Autodesk Inventor part; units mm, degrees
ref_plane "作業平面1" through (14.45, -5.25, 10.5) normal (0, 0, 1) x (0, 1, 0)
ref_plane "YZ Plane" through (0, 0, 0) normal (1, 0, 0) x (0, 1, 0)
ref_plane "XZ Plane" through (0, 0, 0) normal (0, 1, 0) x (-1, 0, 0)
ref_plane "作業平面1" through (14.45, -5.25, 10.5) normal (0, 0, 1) x (0, 1, 0)
sketch "スケッチ1" plane through (14.45, -5.25, 10.5) normal (0, 0, 1) x (0, 1, 0)
  circle A0 centre (4.8, 4.5) radius 1.25
  circle A1 centre (4.8, 14.5) radius 1.25
  circle A2 centre (4.5, 225.5) radius 1.5
  circle A3 centre (4.5, 201.5) radius 1.5
  line L0 (9, 0) -> (0, 0)
  line L1 (9, 0) -> (9, 230)
  line L2 (0, 230) -> (9, 230)
  line L3 (0, 0) -> (0, 230)
  circle A4 centre (-11.4155, 9.5) radius 1.25
  circle A5 centre (4.8, 14.5) radius 4.6
  circle A6 centre (4.8, 4.5) radius 4.6
  circle A7 centre (-11.4155, 9.5) radius 4.25
  line L4 (9.4, 19.1) -> (-15.6655, 19.1)
  line L5 (-15.6655, 19.1) -> (-15.6655, -0.1)
  line L6 (-15.6655, -0.1) -> (9.4, -0.1)
  line L7 (9.4, -0.1) -> (9.4, 19.1)
  point P0 (5.25, 14.45)
  dimension "d0" = 2.5
  dimension "d1" = 9.2
  dimension "d2" = 9.2
  dimension "d3" = 8.5
  dimension "d14" = 2.5
extrude "押し出し1" add sketch "スケッチ1" along normal blind 3 contours L1 A6 L7 L6 L0 | L0 A6 L1 | A6 L0 | L0 A6 L1 | L1 A6 | A7 | A6 L6 L5 L4 L3 L0 | L0 L3 L4 A5 L1 A6 | L1 A5 L7 A6 | A5 L1 | L1 A5 | A5 L1 L4 L7 | A5 L4 L1
sketch "スケッチ2" plane through (14.45, -5.25, 10.5) normal (0, 0, -1) x (-1, 0, 0)
  circle A0 centre (4.5, 4.8) radius 1.25
  circle A1 centre (14.5, 4.8) radius 1.25
  circle A2 centre (9.5, -11.4155) radius 1.25
  line L0 (-0.1, -15.6655) -> (-0.1, 9.4)
  line L1 (-0.1, 9.4) -> (19.1, 9.4)
  line L2 (19.1, 9.4) -> (19.1, -15.6655)
  line L3 (19.1, -15.6655) -> (-0.1, -15.6655)
  circle A3 centre (4.5, 4.8) radius 3
  circle A4 centre (14.5, 4.8) radius 3
  circle A5 centre (9.5, -11.4155) radius 4
  line L4 (4.5, 4.8) -> (9.5, -11.4155) construction
  line L5 (3.0666, 4.358) -> (8.0666, -11.8575)
  line L6 (10.9334, -10.9735) -> (5.9334, 5.242)
  arc A6 (5.9334, 5.242) -> (3.0666, 4.358) centre (4.5, 4.8) ccw
  arc A7 (8.0666, -11.8575) -> (10.9334, -10.9735) centre (9.5, -11.4155) ccw
  line L7 (9.5, -11.4155) -> (14.5, 4.8) construction
  line L8 (10.9334, -11.8575) -> (15.9334, 4.358)
  line L9 (13.0666, 5.242) -> (8.0666, -10.9735)
  arc A8 (8.0666, -10.9735) -> (10.9334, -11.8575) centre (9.5, -11.4155) ccw
  arc A9 (15.9334, 4.358) -> (13.0666, 5.242) centre (14.5, 4.8) ccw
  line L10 (4.5, 4.8) -> (14.5, 4.8) construction
  line L11 (4.5, 3.3) -> (14.5, 3.3)
  line L12 (14.5, 6.3) -> (4.5, 6.3)
  arc A10 (4.5, 6.3) -> (4.5, 3.3) centre (4.5, 4.8) ccw
  arc A11 (14.5, 3.3) -> (14.5, 6.3) centre (14.5, 4.8) ccw
  point P0 (14.45, 5.25)
  point P1 (7, -3.3077)
  point P2 (12, -3.3077)
  point P3 (9.5, 4.8)
  dimension "d6" = 6
  dimension "d7" = 6
  dimension "d8" = 8
  dimension "d9" = 3
  dimension "d10" = 3
  dimension "d11" = 3
extrude "押し出し2" cut sketch "スケッチ2" against normal blind 10 contours A0 | A1 | A2 | A3 L11 L6 A6 L12 | A3 L12 A4 L11 | L12 A6 L5 A3 | A3 L6 L11 | L5 A10 L11 L6 A3 | A3 L6 L9 A5 L5 | L12 A9 L9 L11 A4 | A4 L8 A9 L12 | A6 L6 L11 A10 | L11 L9 A4 | L5 A7 L8 A5 | A5 L9 A8 L5 | A9 A11 L11 L9 | L9 A4 L8 A5 L6 | L6 A5 L9 | L9 L11 A11 L8 A4 | A5 L6 A7 A8 L9 | A5 L8 A7 L6 keep common part
properties part number "従動節固定"
Could you check a few things on this model? Use its own coordinates, in mm. A direction names the side the tool comes from. Coordinates: 2 decimals unless noted, no trailing zeros. Write each loop counter-clockwise with the first axis right and the second up, starting at its lowest first coordinate (ties: lowest second). Pieces come first, ordered by that corner, then holes. Notation, with made-up numbers: (12, 44) -> (20, 44) arc R11 cw to (20, 64) -> close; hole circle Ø4 at (22, 64). An arc over 180 degrees is marked (long way). Return JSON: item names as keys, results as strings.
(1) Imagine slicing it at B-B, the plane z = 13.05. Please give me the cut outline in (x, y), then the cut area to 3 significant figures.
Numbers:
{"outline": "(-0.72, -3.37) -> (2.42, -13.56) arc R4 ccw (long way) to (7.48, -13.56) -> (10.62, -3.37) arc R3 ccw (long way) to (7.35, 1.05) -> (2.55, 1.05) arc R3 ccw (long way) to start; hole circle Ø2.5 at (-0.05, -0.45); hole (2.15, -2.49) -> (4.95, -11.57) -> (7.75, -2.49) arc R3 cw to (7.35, -1.95) -> (2.55, -1.95) arc R3 cw to start; hole circle Ø2.5 at (4.95, -16.67); hole circle Ø2.5 at (9.95, -0.45)", "area": "166 mm2"}
(2) Which directions (+Z, -Z, +X, -X, +Y, -Y) give clear straight access to the entire face, cutting with the end or side of a thin tool? Please do faces 1 (the flat face through (7, -7, 13.5)), 2 (the flat face through (5, -1.95, 12)), 3 (the flat face through (0.875, -8.541, 11.979)), 4 (the flat face through (9.07, -8.4, 11.98)), 5 (the flat face through (7, -7, 10.5)).
Numbers:
{"face 1": "+Z, +X, -X, +Y, -Y", "face 2": "+Z, -Z", "face 3": "+Z, -Z, -X", "face 4": "+Z, -Z, +X", "face 5": "-Z, +X, -X, +Y, -Y"}
(3) Imagine slicing it at A-A, the plane y = -0.45. Please give me the cut outline in (x, z), then the cut area to 3 significant figures.
Numbers:
{"outline": "(-3.05, 10.5) -> (-1.3, 10.5) -> (-1.3, 13.5) -> (-3.05, 13.5) -> close; (1.2, 10.5) -> (8.7, 10.5) -> (8.7, 13.5) -> (1.2, 13.5) -> close; (11.2, 10.5) -> (12.95, 10.5) -> (12.95, 13.5) -> (11.2, 13.5) -> close", "area": "33.0 mm2"}
(4) I'm going to push flat-ended pins straight in: pin 1 (1.5 mm diameter, centred on x = 4.5, z = 11.5, fed in from -Y); pin 2 (1.5 mm diameter, centred on x = 3.5, z = 11.5, fed in from +Y). Where does each tip first touch, or does it pass through?
Numbers:
{"pin 1": "stops at y = -20.67", "pin 2": "stops at y = 1.05"}
(5) Imagine slicing it at C-C, the plane x = 4.25. Please give me the cut outline in (y, z).
Numbers:
{"outline": "(-20.6, 10.5) -> (-17.7, 10.5) -> (-17.7, 13.5) -> (-20.6, 13.5) -> close; (-15.63, 10.5) -> (-9.3, 10.5) -> (-9.3, 13.5) -> (-15.63, 13.5) -> close; (-1.95, 10.5) -> (1.05, 10.5) -> (1.05, 13.5) -> (-1.95, 13.5) -> close"}
(6) We'd pull the mould along Y, two halves only. Please class faces 6 (the flat face through (5, 1.05, 12)), 7 (the cylindrical face through (5.088, -20.663, 11.979)), 8 (the cylindrical face through (12.31, 1.4, 11.98)): +Y half, -Y half, draft (parallel to the pull), parting line (faces both ways), or undercut.
Numbers:
{"face 6": "+Y half", "face 7": "undercut", "face 8": "parting line"}
(7) I need wall thicknesses on L1, parallel to X at y = -0.45, z = 11.3; L2, parallel to X at y = 0, z = 12.35; L3, parallel to X at y = -9.25, z = 11. Which ranges of each line are inside material? Lowest first, please.
Numbers:
{"L1": "x = -3.05 to -1.3, 1.2 to 8.7, 11.2 to 12.95", "L2": "x = -3.02 to -1.22, 1.12 to 8.78, 11.12 to 12.92", "L3": "x = 1.09 to 4.23, 5.67 to 8.81"}
(8) Imagine slicing it at D-D, the plane y = -4.5. Please give me the cut outline in (x, z), then the cut area to 3 significant figures.
Numbers:
{"outline": "(-0.37, 10.5) -> (2.77, 10.5) -> (2.77, 13.5) -> (-0.37, 13.5) -> close; (7.13, 10.5) -> (10.27, 10.5) -> (10.27, 13.5) -> (7.13, 13.5) -> close", "area": "18.8 mm2"}
